```python
from build123d import *

# Parameters (mm, degrees)
F1_DEPTH = 31.75
F3_DEPTH = 12.7
F5_DEPTH = 12.7
F7_DEPTH = 12.7


with BuildPart() as f1:
    # F0 (on Top) → F1 (new body)
    with BuildSketch(Plane.XY):
        Polygon((0, 31.75), (0, 0), (38.1, 0), (38.1, 31.75), (25.4, 31.75), (25.4, 57.15), (12.7, 57.15), (12.7, 31.75), align=None)
    extrude(amount=F1_DEPTH)

    # F2 (on face) → F3 (cut)
    with BuildSketch(Plane(origin=(0, 0, 0), x_dir=(0, -1, 0), z_dir=(-1, 0, 0))):
        Polygon((-31.75, 31.75), (-31.75, 0), (-19.05, 31.75), align=None)
    extrude(amount=-F3_DEPTH, mode=Mode.SUBTRACT)

    # F4 (on face) → F5 (cut)
    with BuildSketch(Plane.YZ.offset(38.1)):
        Polygon((19.05, 31.75), (31.75, 0), (31.75, 31.75), align=None)
    extrude(amount=-F5_DEPTH, mode=Mode.SUBTRACT)

    # F6 (on face) → F7 (cut)
    with BuildSketch(Plane.YZ.offset(25.4)):
        Polygon((57.15, 0), (57.15, 31.75), (44.45, 31.75), align=None)
    extrude(amount=-F7_DEPTH, mode=Mode.SUBTRACT)


solid = f1.part
```
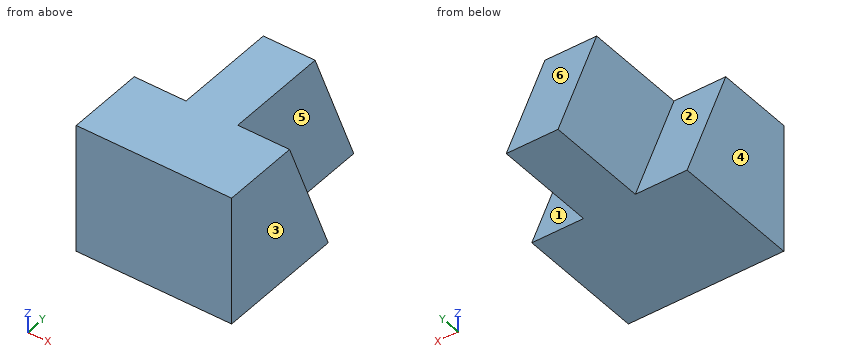
Build history of the part. All positions in model axes, mm. Face numbers are marked on the shaded views. A direction names the side the tool comes from. Give positions to 0.01 mm unless a question says otherwise; leave off trailing zeros. Order: outer loops, then holes, each group sorted by start corner. A loop starts at its lowest first (then second) coordinate and runs counter-clockwise, first axis right, second up. Notation, with made-up numbers: M 73.5,55 L 92.5,55 A16 cw 92.5,84 Z; hole C -24.75,20 d2. An arc over 180 degrees is marked long. Return JSON: item names as keys, results as strings.
Q1. Wall check: probe 1 along X at (y, z) = (42.5, 17.5); probe 2 along Y at (x, z) = (10.5, 26); probe 3 along Y at (x, z) = (23, 11). Give the ranges that are in metal, low to high. Write a range as from..to.
Answer list:
{"probe 1": "x = 12.7..25.4", "probe 2": "y = 0..21.35", "probe 3": "y = 0..52.75"}
Q2. Band-saw the part on C-C (x = 15.5). Give the cut face in (y, z).
Answer list:
{"outline": "M 0,0 L 57.15,0 L 44.45,31.75 L 0,31.75 Z"}
Q3. Band-saw the part on D-D (x = 27). Give the cut face in (y, z), then the cut area to 3 significant figures.
Answer list:
{"outline": "M 0,0 L 31.75,0 L 19.05,31.75 L 0,31.75 Z", "area": "806 mm^2"}
Q4. Two-plate mould, pull along X, no slides. Class the marked faces 4, 5 and 6: pulls with the +X half, pulls with the -X half, needs draft (parallel to the pull), parting line crosses it, or undercut.
Answer list:
{"face 4": "pulls with the -X half", "face 5": "pulls with the +X half", "face 6": "needs draft"}
Q5. Band-saw the part on A-A (z = 25.5). Give the cut face in (x, y), then the cut area to 3 significant figures.
Answer list:
{"outline": "M 0,0 L 38.1,0 L 38.1,21.55 L 25.4,21.55 L 25.4,46.95 L 12.7,46.95 L 12.7,21.55 L 0,21.55 Z", "area": "1,140 mm^2"}
Q6. 3-axis set-ups, long thin cutter, end or side, ignore diameter. For the marked faces 1, 2 and 3: which of +Z, -Z, +X, -X, +Y, -Y reach the whole face in a straight line?
Answer list:
{"face 1": "+Z, +X, +Y", "face 2": "+Z, -X, +Y", "face 3": "+Z, -Z, +X, +Y, -Y"}
Q7. Flat gauge pins, fed straight in: pin 1 (1 mm diameter, centred on x = 9, z = 9.5, fed in from +Y); pin 2 (8 mm diameter, centred on y = 50.5, z = 8, fed in from -X); pin 3 (16 mm diameter, centred on y = 44.5, z = 23, fed in from +X). Where does each tip first touch, or does it go through?
Answer list:
{"pin 1": "stops at y = 28.15", "pin 2": "stops at x = 12.7", "pin 3": "stops at x = 25.4"}
Q8. Band-saw the part on B-B (y = 21). Give the cut face in (x, z) (3 decimals), then the cut area to 3 significant figures.
Answer list:
{"outline": "M 0,0 L 38.1,0 L 38.1,26.875 L 25.4,26.875 L 25.4,31.75 L 12.7,31.75 L 12.7,26.875 L 0,26.875 Z", "area": "1,090 mm^2"}
